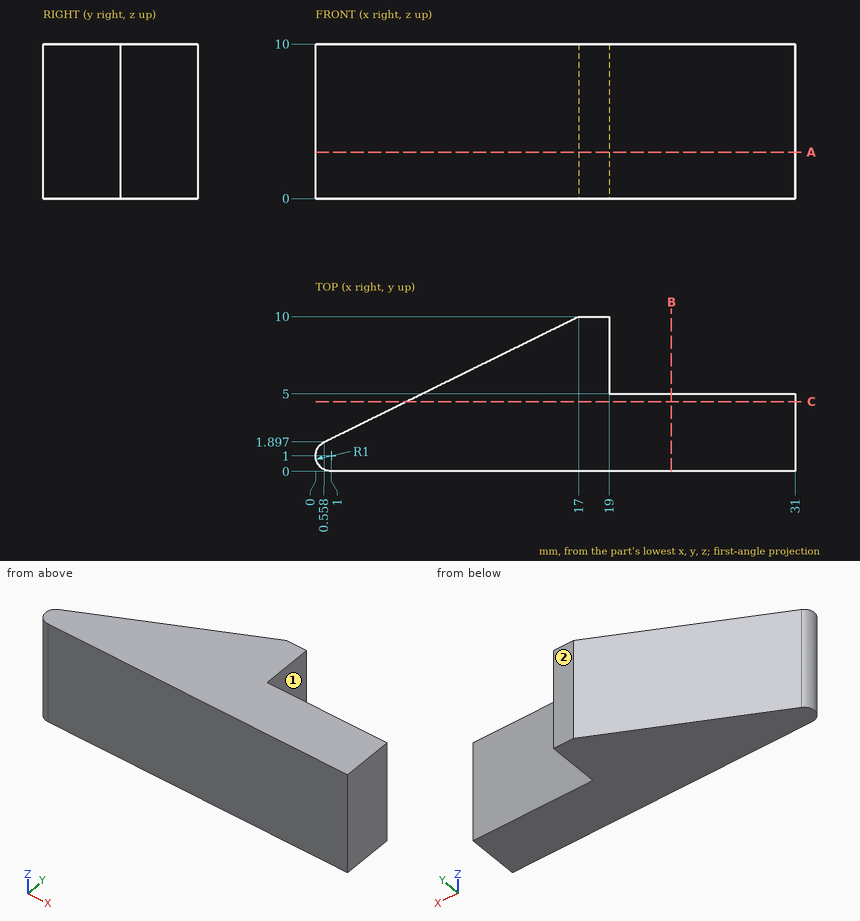
Here's the drawing with two shaded views (mm, measured from the low corner). I have some questions. A direction names the side the tool comes from. Give positions to 0.01 mm unless a question says otherwise; leave off trailing zeros. Loops run counter-clockwise (first coordinate to the right, second up) from the corner with the lowest first, then second, coordinate; pieces in that order, holes last. Notation, with made-up numbers: M -24,84 L 10,84 A28 cw 10,116 Z; hole C -29.5,-12.5 d2. An arc over 180 degrees is marked long. One line per item, written item: value.
(1) Will these pins go through, and if not, where does the flat tip stop? pin 1 (3 mm diameter, centred on x = 24.5, z = 4, fed in from +Y); pin 2 (2.5 mm diameter, centred on y = 8.5, z = 5, fed in from +X); pin 3 (6 mm diameter, centred on y = 2, z = 6, fed in from -X).
Returned:
pin 1: y = 5
pin 2: x = 19
pin 3: x = 0
(2) Suppose I cut it at B-B on x = 23. List the corners of the cut face in (y, z) for me.
Returned:
outline: M 0,0 L 5,0 L 5,10 L 0,10 Z
(3) Suppose I cut it at C-C on y = 4.5. List the corners of the cut face in (x, z) for me, plus the area to 3 significant figures.
Returned:
outline: M 5.84,0 L 31,0 L 31,10 L 5.84,10 Z
area: 252 mm^2
(4) Which directions (+Z, -Z, +X, -X, +Y, -Y) give clear straight access to the entire face, cutting with the end or side of a thin tool? Please do the marked faces 1 and 2.
Returned:
face 1: +Z, -Z, +X, +Y
face 2: +Z, -Z, +X, -X, +Y
(5) Suppose I cut it at A-A on z = 3. List the corners of the cut face in (x, y) for me.
Returned:
outline: M 0.56,1.9 A1 ccw 1,0 L 31,0 L 31,5 L 19,5 L 19,10 L 17,10 Z
(6) I need wall thicknesses on line 1 (Y direction, x = 25, z = 9.75); line 2 (X direction, y = 8, z = 8.25); line 3 (X direction, y = 5.25, z = 7.25). Which ranges of each line are inside material? Lowest first, please.
Returned:
line 1: 0 to 5
line 2: 12.94 to 19
line 3: 7.36 to 19
